from build123d import *

# Parameters (mm, degrees)
F1_DEPTH = 63.5
F2_DEPTH = 25.4
F3_DEPTH = 7.9375
F0_W     = 53.001129165
F0_H     = 29.8131351553
F5_R     = 6.35


with BuildPart() as f1:
    # F0 (on Front) → F1 (new body, symmetric)
    with BuildSketch(Plane.XZ):
        Polygon((22.225, 9.525), (-41.275, 9.525), (-41.275, -9.525), (41.275, -9.525), (41.275, 9.525), align=None)
    extrude(amount=F1_DEPTH, both=True)

    # F0 (on Front) → F2 (join, symmetric)
    with BuildSketch(Plane.XZ):
        with BuildLine():
            Line((22.225, 61.9252), (22.225, 9.525))
            Line((22.225, 9.525), (41.275, 9.525))
            Line((41.275, 9.525), (41.275, 61.9252))
            ThreePointArc((41.275, 61.9252), (45.9246798487, 73.1505201513), (57.15, 77.8002))
            Line((57.15, 77.8002), (74.9244145172, 77.8002))
            Line((74.9244145172, 77.8002), (74.9244145172, 96.8502))
            Line((74.9244145172, 96.8502), (57.15, 96.8502))
            add(Edge.make_bspline(
                [(47.222675354, 95.4095821859), (50.4096853914, 95.9076958448), (53.7170651414, 96.3865930832), (57.15, 96.8502)],
                knots=[125.3666616532, 125.3666616532, 125.3666616532, 125.3666616532, 131.5795241671, 131.5795241671, 131.5795241671, 131.5795241671], degree=3))
            ThreePointArc((47.222675354, 95.4095821859), (29.1636869322, 82.8183066591), (22.225, 61.9252))
        make_face()
    extrude(amount=F2_DEPTH, both=True)

    # F0 (on Front) → F3 (join, symmetric)
    with BuildSketch(Plane.XZ):
        with BuildLine():
            add(Edge.make_bspline(
                [(-41.275, 9.525), (-32.3844300355, 67.4827050573), (-17.0866197814, 85.3583624135), (47.222675354, 95.4095821859)],
                knots=[0, 0, 0, 0, 125.3666616532, 125.3666616532, 125.3666616532, 125.3666616532], degree=3))
            Line((-41.275, 9.525), (22.225, 9.525))
            Line((22.225, 9.525), (22.225, 61.9252))
            ThreePointArc((22.225, 61.9252), (29.1636869322, 82.8183066591), (47.222675354, 95.4095821859))
        make_face()
    extrude(amount=F3_DEPTH, both=True)

    # F0 (on Front) → F4 (revolve)
    with BuildSketch(Plane.XZ):
        with Locations((101.560038097, 86.7887464721)):
            Rectangle(F0_W, F0_H)
    revolve(axis=Axis((75.0594735146, 0, 86.7887464721), (0, 0, 1)))

    # F5
    f5_edges = [f1.edges().sort_by_distance(p)[0] for p in [
        (41.275, -63.5, 0),
        (-41.275, -63.5, 0),
        (41.275, 63.5, 0),
        (-41.275, 63.5, 0),
    ]]
    fillet(f5_edges, radius=F5_R)


solid = f1.part
Part model, mm, in its own coordinate system. A direction names the side the tool comes from. Round coordinates to 2 decimals unless told otherwise and drop trailing zeros. Write each loop counter-clockwise with the first axis right and the second up, starting at its lowest first coordinate (ties: lowest second). Pieces come first, ordered by that corner, then holes. Notation, with made-up numbers: M 70,73 L 91,73 A13 ccw 91,81 Z; hole C 43,16 d10. An arc over 180 degrees is marked long. Return JSON: item names as keys, results as strings. Group by question number.
(1) Saw through at A-A on z = 0.5. Write the cut outline in (x, y) (3 decimals).
(2) Saw through at D-D on y = 15. Write the cut outline in (x, z) (3 decimals).
(3) Which spindle directions (+Z, -Z, +X, -X, +Y, -Y) get a long thin tool onto all of the face, cutting with end or side? Do faces 1 (the face through (22.225, 17, 36)), 2 (the face through (39.464, -61.59, 0.133)), 3 (the face through (22.225, -17, 36)), 4 (the face through (124.02, -20.3, 87)). Say none if no direction does.
(4) Pin check, flat tips, straight feed: pin 1 Ø8 at (y, z) = (-9, 34) entering from +X (3 decimals); pin 2 Ø11.5 at (x, z) = (31, 59) entering from +Y; pin 3 Ø18 at (x, z) = (35.5, 54) entering from -Y; pin 4 Ø3 at (y, z) = (-27.5, 33) entering from +X. Stop position of each tip, or through.
(5) Drill centre lines: probe 1 along Z at (x, y) = (34, -27) (3 decimals); probe 2 along Y at (x, z) = (37, 64.5); probe 3 along Z at (x, y) = (8.5, -16) (3 decimals). Where is each one in solid material? Low to high.
(6) Saw through at B-B on y = -46.5. Write the cut outline in (x, z) (3 decimals).
(7) Saw through at C-C on x = 39. Write the cut outline in (y, z) (3 decimals).
Returned:
{
 "1": {"outline": "M -41.275,-57.15 A6.35 ccw -34.925,-63.5 L 34.925,-63.5 A6.35 ccw 41.275,-57.15 L 41.275,57.15 A6.35 ccw 34.925,63.5 L -34.925,63.5 A6.35 ccw -41.275,57.15 Z"},
 "2": {"outline": "M -41.275,-9.525 L 41.275,-9.525 L 41.275,61.925 A15.875 cw 44.786,71.882 L 125.894,71.882 L 125.894,101.695 L 24.225,101.695 L 24.225,73.575 A34.925 ccw 22.225,61.925 L 22.225,9.525 L -41.275,9.525 Z"},
 "3": {"face 1": "+Z, -X, +Y", "face 2": "+Z, -Z, +X, -Y", "face 3": "+Z, -X, -Y", "face 4": "+Z"},
 "4": {"pin 1": "x = 41.275", "pin 2": "y = 25.4", "pin 3": "y = -25.4", "pin 4": "through"},
 "5": {"probe 1": "-9.525 to 9.525, 71.882 to 101.695", "probe 2": "-25.4 to 25.4", "probe 3": "-9.525 to 9.525"},
 "6": {"outline": "M -41.275,-9.525 L 41.275,-9.525 L 41.275,9.525 L -41.275,9.525 Z; M 49.626,71.882 L 100.493,71.882 L 100.493,101.695 L 49.626,101.695 Z"},
 "7": {"outline": "M -62.02,-9.525 L 62.02,-9.525 L 62.02,9.525 L 25.4,9.525 L 25.4,71.882 L 38.844,71.882 L 38.844,101.695 L -38.844,101.695 L -38.844,71.882 L -25.4,71.882 L -25.4,9.525 L -62.02,9.525 Z"}
}
